Part print with two shaded views. Sizes in mm from the minimum x, y, z corner. Coordinates: 2 decimals unless noted, no trailing zeros. Loops run counter-clockwise (first coordinate to the right, second up) from the corner with the lowest first, then second, coordinate; pieces in that order, holes last.
Item 1: Cut at B-B (y = 8.75). List the corners of the cut face in (x, z).
Item 2: Flat gauge pins, fed straight in: pin 1 (10 mm diameter, centred on x = 17, y = 4.5, fed in from -Z); pin 2 (1.5 mm diameter, centred on x = 15.5, z = 2, fed in from -Y). Where does each tip first touch, or does it go through?
Item 3: Mould opens along X. For the marked faces 1, 2, 3 and 4 say: released by +X, released by -X, zero draft, split by the parting line, or undercut.
Item 4: Cut at C-C (z = 0.5). List the corners of the cut face in (x, y), and give its area (3 significant figures).
Item 5: Cut at A-A (x = 10). List the corners of the cut face in (y, z), and give its area (3 significant figures).
Item 6: Cut at D-D (y = 5.75). List the corners of the cut face in (x, z).
Item 7: Drill centre lines: line 1 along X through (y, z) = (6, 0.65) (1 decimal); line 2 along X through (y, z) = (9, 1.2); line 3 along X through (y, z) = (8, 0.9) (1 decimal). Where is each one in solid material? Low to high.
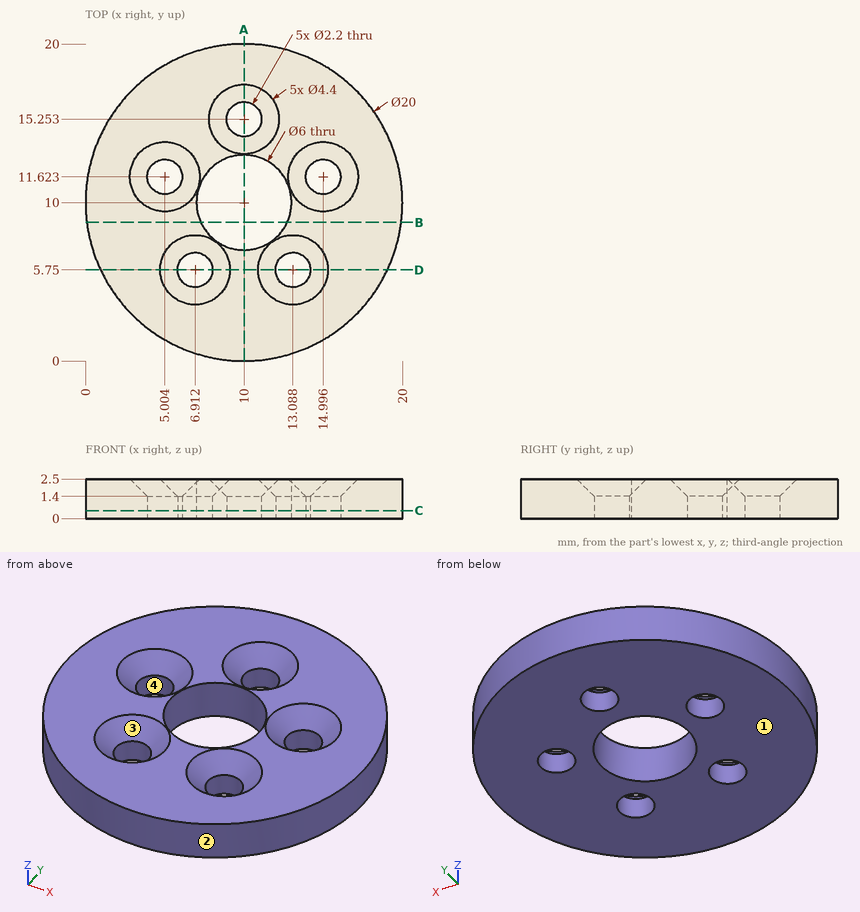
Filled sheet:
1. outline: (0.08, 0) - (7.27, 0) - (7.27, 2.5) - (0.08, 2.5) - close; (12.73, 0) - (19.92, 0) - (19.92, 2.5) - (12.73, 2.5) - close
2. pin 1: stops at z = 0
2. pin 2: stops at y = 1.2
3. face 1: zero draft
3. face 2: split by the parting line
3. face 3: undercut
3. face 4: undercut
4. outline: circle Ø20 at (10, 10); hole circle Ø2.2 at (5, 11.62); hole circle Ø2.2 at (6.91, 5.75); hole circle Ø6 at (10, 10); hole circle Ø2.2 at (10, 15.25); hole circle Ø2.2 at (13.09, 5.75); hole circle Ø2.2 at (15, 11.62)
4. area: 267 mm2
5. outline: (0, 0) - (7, 0) - (7, 2.5) - (0, 2.5) - close; (13, 0) - (14.15, 0) - (14.15, 1.4) - (13.05, 2.5) - (13, 2.5) - close; (16.35, 0) - (20, 0) - (20, 2.5) - (17.45, 2.5) - (16.35, 1.4) - close
5. area: 28.3 mm2
6. outline: (0.95, 0) - (5.81, 0) - (5.81, 1.4) - (4.71, 2.5) - (0.95, 2.5) - close; (8.01, 0) - (11.99, 0) - (11.99, 1.4) - (10.89, 2.5) - (9.11, 2.5) - (8.01, 1.4) - close; (14.19, 0) - (19.05, 0) - (19.05, 2.5) - (15.29, 2.5) - (14.19, 1.4) - close
7. line 1: x = 0.8 to 5.8, 8 to 12, 14.2 to 19.2
7. line 2: x = 0.05 to 7.17, 12.83 to 19.95
7. line 3: x = 0.2 to 7.8, 12.2 to 19.8
